Geometry: final body of the model. Coordinates: model frame, mm. Give positions to 0.01 mm unless a question says otherwise; leave off trailing zeros. Loops run counter-clockwise (first coordinate to the right, second up) from the corner with the lowest first, then second, coordinate; pieces in that order, holes last. Notation, with made-up numbers: (25, -1.75) - (58, -1.75) arc R31 cw to (58, 27.25) - close; hole circle Ø3 at (-26.75, 86.25). An arc over 180 degrees is marked (long way). Use one line per item in the form item = value.
```python
from build123d import *

# Parameters (mm, degrees)
SKETCH3_W           = 234.95
SKETCH3_H           = 30.48
SKETCH3_R           = 1.574999898
SKETCH3_W_2         = 25.4
SKETCH3_H_2         = 3.175
BOSS_EXTRUDE1_DEPTH = 3.175
SKETCH4_W           = 107.95
SKETCH4_H           = 3.175
SKETCH4_W_2         = 12.7
BOSS_EXTRUDE2_DEPTH = 3.175
SKETCH5_W           = 3.175
SKETCH5_H           = 17.78
SKETCH5_W_2         = 3.81
CUT_EXTRUDE1_DEPTH  = 7.62


with BuildPart() as part:
    # Sketch3 → Boss-Extrude1 (new body)
    # profile 1 of 7: a face of its own
    with BuildSketch(Plane.XY):
        with Locations((-63.5, 8.8475)):
            Rectangle(SKETCH3_W, SKETCH3_H)
        with BuildLine():
            ThreePointArc((-163.6, 17.5), (-162.135533906, 21.035533906), (-158.6, 22.5))
            Line((-158.6, 22.5), (-127, 22.5))
            Line((-127, 22.5), (-101.6, 22.5))
            Line((-101.6, 22.5), (-101.6, 19.325))
            Line((-101.6, 19.325), (-101.6, 3.175))
            Line((-101.6, 3.175), (-101.6, 0))
            Line((-101.6, 0), (-127, 0))
            Line((-127, 0), (-158.6, 0))
            ThreePointArc((-158.6, 0), (-162.135533906, 1.464466094), (-163.6, 5))
            Line((-163.6, 5), (-163.6, 17.5))
        make_face(mode=Mode.SUBTRACT)
        with BuildLine():
            Line((-25.4, 22.5), (0, 22.5))
            Line((0, 22.5), (31.6, 22.5))
            ThreePointArc((31.6, 22.5), (35.135533906, 21.035533906), (36.6, 17.5))
            Line((36.6, 17.5), (36.6, 5))
            ThreePointArc((36.6, 5), (35.135533906, 1.464466094), (31.6, 0))
            Line((31.6, 0), (0, 0))
            Line((0, 0), (-25.4, 0))
            Line((-25.4, 0), (-25.4, 3.175))
            Line((-25.4, 3.175), (-25.4, 19.325))
            Line((-25.4, 19.325), (-25.4, 22.5))
        make_face(mode=Mode.SUBTRACT)
    # profile 2 of 7: a face of its own
    with BuildSketch(Plane.XY):
        with BuildLine():
            ThreePointArc((-158.6, 0), (-162.135533906, 1.464466094), (-163.6, 5))
            Line((-163.6, 5), (-163.6, 17.5))
            ThreePointArc((-163.6, 17.5), (-162.135533906, 21.035533906), (-158.6, 22.5))
            Line((-158.6, 22.5), (-127, 22.5))
            Line((-127, 22.5), (-127, 0))
            Line((-127, 0), (-158.6, 0))
        make_face()
        with Locations((-132.45, 20.25)):
            Circle(SKETCH3_R, mode=Mode.SUBTRACT)
        with Locations((-132.45, 2.250000072)):
            Circle(SKETCH3_R, mode=Mode.SUBTRACT)
        with BuildLine():
            ThreePointArc((-143.175, 11.25), (-141.3, 13.125), (-139.425, 11.25))
            ThreePointArc((-139.425, 11.25), (-141.3, 9.375), (-143.175, 11.25))
        make_face(mode=Mode.SUBTRACT)
        with BuildLine():
            ThreePointArc((-155.35, 11.25), (-152.6, 14), (-149.85, 11.25))
            ThreePointArc((-149.85, 11.25), (-152.6, 8.5), (-155.35, 11.25))
        make_face(mode=Mode.SUBTRACT)
    # profile 3 of 7: a face of its own
    with BuildSketch(Plane.XY):
        with BuildLine():
            Line((36.6, 5), (36.6, 17.5))
            ThreePointArc((36.6, 17.5), (35.135533906, 21.035533906), (31.6, 22.5))
            Line((31.6, 22.5), (0, 22.5))
            Line((0, 22.5), (0, 0))
            Line((0, 0), (31.6, 0))
            ThreePointArc((31.6, 0), (35.135533906, 1.464466094), (36.6, 5))
        make_face()
        with Locations((5.45, 2.250000072)):
            Circle(SKETCH3_R, mode=Mode.SUBTRACT)
        with Locations((5.45, 20.25)):
            Circle(SKETCH3_R, mode=Mode.SUBTRACT)
        with BuildLine():
            ThreePointArc((16.175, 11.25), (14.3, 13.125), (12.425, 11.25))
            ThreePointArc((12.425, 11.25), (14.3, 9.375), (16.175, 11.25))
        make_face(mode=Mode.SUBTRACT)
        with BuildLine():
            ThreePointArc((28.35, 11.25), (25.6, 14), (22.85, 11.25))
            ThreePointArc((22.85, 11.25), (25.6, 8.5), (28.35, 11.25))
        make_face(mode=Mode.SUBTRACT)
    # profile 4 of 7: a face of its own
    with BuildSketch(Plane.XY):
        with Locations((-12.7, 1.5875)):
            Rectangle(SKETCH3_W_2, SKETCH3_H_2)
    # profile 5 of 7: a face of its own
    with BuildSketch(Plane.XY):
        with Locations((-12.7, 20.9125)):
            Rectangle(SKETCH3_W_2, SKETCH3_H_2)
    # profile 6 of 7: a face of its own
    with BuildSketch(Plane.XY):
        with Locations((-114.3, 20.9125)):
            Rectangle(SKETCH3_W_2, SKETCH3_H_2)
    # profile 7 of 7: a face of its own
    with BuildSketch(Plane.XY):
        with Locations((-114.3, 1.5875)):
            Rectangle(SKETCH3_W_2, SKETCH3_H_2)
    extrude(amount=BOSS_EXTRUDE1_DEPTH)

    # Sketch4 → Boss-Extrude2 (add)
    with BuildSketch(Plane.XY.offset(3.175)):
        with Locations((-63.5, 28.85)):
            Rectangle(SKETCH4_W, SKETCH4_H)
        with Locations((-136.525, 28.85)):
            Rectangle(SKETCH4_W_2, SKETCH4_H)
        with Locations((-161.925, 28.85)):
            Rectangle(SKETCH4_W_2, SKETCH4_H)
        Polygon((-142.875, 27.2625), (-155.575, 27.2625), (-168.275, 27.2625), (-180.975, 27.2625), (-180.975, 24.0875), (53.975, 24.0875), (53.975, 27.2625), (41.275, 27.2625), (28.575, 27.2625), (15.875, 27.2625), (3.175, 27.2625), (-9.525, 27.2625), (-117.475, 27.2625), (-130.175, 27.2625), align=None)
        with Locations((9.525, 28.85)):
            Rectangle(SKETCH4_W_2, SKETCH4_H)
        with Locations((34.925, 28.85)):
            Rectangle(SKETCH4_W_2, SKETCH4_H)
        Polygon((53.975, -6.3925), (-180.975, -6.3925), (-180.975, -9.5675), (-168.275, -9.5675), (-155.575, -9.5675), (-142.875, -9.5675), (-130.175, -9.5675), (-117.475, -9.5675), (-9.525, -9.5675), (3.175, -9.5675), (15.875, -9.5675), (28.575, -9.5675), (41.275, -9.5675), (53.975, -9.5675), align=None)
        with Locations((34.925, -11.155)):
            Rectangle(SKETCH4_W_2, SKETCH4_H)
        with Locations((9.525, -11.155)):
            Rectangle(SKETCH4_W_2, SKETCH4_H)
        with Locations((-63.5, -11.155)):
            Rectangle(SKETCH4_W, SKETCH4_H)
        with Locations((-136.525, -11.155)):
            Rectangle(SKETCH4_W_2, SKETCH4_H)
        with Locations((-161.925, -11.155)):
            Rectangle(SKETCH4_W_2, SKETCH4_H)
    extrude(amount=-BOSS_EXTRUDE2_DEPTH)

    # Sketch5 → Cut-Extrude1 (cut)
    with BuildSketch(Plane.XY.offset(3.175)):
        with Locations((-179.3875, 8.8475)):
            Rectangle(SKETCH5_W, SKETCH5_H)
        with Locations((52.07, 8.8475)):
            Rectangle(SKETCH5_W_2, SKETCH5_H)
    extrude(amount=-CUT_EXTRUDE1_DEPTH, mode=Mode.SUBTRACT)


solid = part.part
```
(1) Cut plane B-B (z = 1). Give the number of separate pieces and of enclosed holes in the cut face, plus the area to 3 significant figures.
Solution:
separate_pieces = 1
enclosed_holes = 10
area = 8,620 mm2
(2) Pull-direction query (Y, two-part tool) for faces 1 (the face through (-65, 9, 3.175)), 2 (the face through (-149.98, 10.42, 1.57)); classes: released by +Y, released by -Y, zero draft, split by the parting line, or undercut.
Solution:
face_1 = zero draft
face_2 = undercut
(3) Cut plane A-A (x = -152.6). Return the cut outline in (y, z) (1 decimal).
Solution:
outline = (-9.6, 0) - (8.5, 0) - (8.5, 3.2) - (-9.6, 3.2) - close; (14, 0) - (27.3, 0) - (27.3, 3.2) - (14, 3.2) - close
(4) Pin query (flat end, axial travel): P1, Ø1, axis at y = 9.5, z = 1, coming from the +X side (3 decimals); P2, Ø1, axis at x = -121, z = 2.5, coming from the +Y side; P3, Ø1, axis at y = 29, z = 1, coming from the +X side (3 decimals). Return the tip coordinate at first contact, or that it passes through.
Solution:
P1 = 50.165
P2 = 27.26
P3 = 41.275
(5) Material intervals for L1, parallel to X at y = 2, z = 1.8 (3 decimals); L2, parallel to X at y = -10, z = 0.2 (3 decimals); L3, parallel to Y at x = -132.45, z = 1.2 (1 decimal), sorted ascending. Write a range as from..to.
Solution:
L1 = -177.8..-134.005, -130.895..3.895, 7.005..50.165
L2 = -168.275..-155.575, -142.875..-130.175, -117.475..-9.525, 3.175..15.875, 28.575..41.275
L3 = -12.7..0.7, 3.8..18.7, 21.8..30.4
